Autodesk Inventor part; units mm, degrees
ref_plane "YZ Plane" through (0, 0, 0) normal (1, 0, 0) x (0, 1, 0)
ref_plane "XZ Plane" through (0, 0, 0) normal (0, 1, 0) x (-1, 0, 0)
ref_plane "XY Plane" through (0, 0, 0) normal (0, 0, 1) x (1, 0, 0)
sketch "Sketch1" plane through (0, 0, 0) normal (0, 0, 1) x (1, 0, 0)
  circle A0 centre (0, 0) radius 22.5
extrude "Extrusion1" add sketch "Sketch1" along normal blind 12
sketch "Sketch2" plane through (0, 0, 12) normal (0, 0, 1) x (1, 0, 0)
  circle A0 centre (0, 0) radius 18
extrude "Extrusion2" add sketch "Sketch2" along normal blind 12
sketch "Sketch3" plane through (0, 0, 24) normal (0, 0, 1) x (1, 0, 0)
  circle A0 centre (0, 0) radius 22.5
extrude "Extrusion3" add sketch "Sketch3" along normal blind 20
sketch "Sketch4" plane through (0, 0, 44) normal (0, 0, 1) x (1, 0, 0)
  circle A0 centre (0, 0) radius 35
extrude "Extrusion4" add sketch "Sketch4" along normal blind 36
sketch "Sketch5" plane through (0, 0, 80) normal (0, 0, 1) x (1, 0, 0)
  circle A0 centre (0, 0) radius 25
extrude "Extrusion5" cut sketch "Sketch5" against normal blind 15
sketch "Sketch6" plane through (0, 0, 80) normal (0, 0, 1) x (1, 0, 0)
  circle A0 centre (0, 0) radius 35
  line L0 (0, 0) -> (-32.4578, -13.0955)
  line L1 (0, 0) -> (-32.4578, 13.0955)
  arc A1 (-32.4578, 13.0955) -> (-32.4578, -13.0955) centre (0, 0) ccw
  line L2 (0, 0) -> (27.5699, -21.5615)
  line L3 (0, 0) -> (4.8879, -34.657)
  arc A2 (4.8879, -34.657) -> (27.5699, -21.5615) centre (0, 0) ccw
  line L4 (0, 0) -> (4.8879, 34.657)
  line L5 (0, 0) -> (27.5699, 21.5615)
  arc A3 (27.5699, 21.5615) -> (4.8879, 34.657) centre (0, 0) ccw
  dimension "d17" = 360
extrude "Extrusion6" cut sketch "Sketch6" against normal blind 15 contours L5 L4 A0 | A0 L3 L2 | L0 A0 L1
sketch "Sketch7" plane through (0, 0, 65) normal (0, 0, 1) x (1, 0, 0)
  arc A0 (11.4564, 5) -> (11.4564, -5) centre (0, 0) ccw
  line L0 (18.8783, 0) -> (18.8783, 5)
  line L1 (18.8783, 0) -> (18.8783, -5)
  line L2 (18.8783, -5) -> (11.4564, -5)
  line L3 (18.8783, 5) -> (11.4564, 5)
extrude "Extrusion7" cut sketch "Sketch7" against normal blind 16
sketch "Sketch8" plane through (0, 0, 0) normal (0, 0, -1) x (-1, 0, 0)
  point P0 (0, 0)
sketch "Sketch9" plane through (0, 0, 49) normal (0, 0, 1) x (1, 0, 0)
  circle A0 centre (0, 0) radius 11.9112
extrude "Extrusion8" cut sketch "Sketch9" against normal blind 50.8
properties part number "tarea 3 dinamica" material "Iron, Ductile"
Part model, mm, in its own coordinate system. A direction names the side the tool comes from. Give positions to 0.01 mm unless a question says otherwise; leave off trailing zeros. Loops run counter-clockwise (first coordinate to the right, second up) from the corner with the lowest first, then second, coordinate; pieces in that order, holes last. Notation, with made-up numbers: (73.5, 36.25) -> (126.5, 36.25) arc R18 cw to (126.5, 65.25) -> close; hole circle Ø9 at (-32.5, 88). An arc over 180 degrees is marked (long way). Write each question's results on one line, items separated by ' | '. Start each with the question number.
Q1. Which spindle directions (+Z, -Z, +X, -X, +Y, -Y) get a long thin tool onto all of the face, cutting with end or side? Do faces 1 (the face through (-12.298, 21.766, 72.605)), 2 (the face through (23.58, -18.44, 72.6)), 3 (the face through (4.18, -29.64, 72.6)). Say none if no direction does.
Q2. Band-saw the part on C-C on z = 54. List the corners of the cut face in (x, y).
Q3. Band-saw the part on A-A on x = 0. List the corners of the cut face in (y, z).
Q4. Wall check: L1, parallel to Y at x = 0, z = 56.25; L2, parallel to Z at x = 14, y = -17; L3, parallel to Y at x = 0, z = 20. Give the ranges that are in metal, low to high.
Q5. Pull direction X, two halves, no side cores. Call faces 4 (the face through (10.382, 19.961, 33.86)), 5 (the face through (-10.1, 15.1, 24)), 6 (the face through (12.4, 0.1, 49)), 7 (the face through (4.18, 29.64, 72.6)): +X half, -X half, draft (parallel to the pull), parting line (faces both ways), or undercut.
Q6. Pin check, flat tips, straight feed: P1, Ø21.5, axis at x = 0, y = 0, coming from the +Z side; P2, Ø12, axis at y = 18.5, z = 41.5, coming from the +X side; P3, Ø1, axis at x = 12, z = 49, coming from the +Y side; P4, Ø2, axis at x = 15, z = 56.5, coming from the +Y side. Stop position of each tip, or through.
Q7. Band-saw the part on D-D on z = 69. List the corners of the cut face in (x, y) (1 decimal), plus the area to 3 significant figures.
Q8. Band-saw the part on B-B on y = 0. List the corners of the cut face in (x, z).
Results are:
1) face 1: +Z | face 2: +Z, -Y | face 3: +Z, +X
2) outline: circle Ø70 at (0, 0); hole (11.46, -5) -> (18.88, -5) -> (18.88, 5) -> (11.46, 5) arc R12.5 ccw (long way) to start
3) outline: (-35, 44) -> (-22.5, 44) -> (-22.5, 24) -> (-18, 24) -> (-18, 12) -> (-22.5, 12) -> (-22.5, 0) -> (-11.91, 0) -> (-11.91, 49) -> (-12.5, 49) -> (-12.5, 65) -> (-25, 65) -> (-25, 80) -> (-35, 80) -> close; (11.91, 0) -> (22.5, 0) -> (22.5, 12) -> (18, 12) -> (18, 24) -> (22.5, 24) -> (22.5, 44) -> (35, 44) -> (35, 80) -> (25, 80) -> (25, 65) -> (12.5, 65) -> (12.5, 49) -> (11.91, 49) -> close
4) L1: y = -35 to -12.5, 12.5 to 35 | L2: z = 0 to 12, 24 to 65 | L3: y = -18 to -11.91, 11.91 to 18
5) face 4: parting line | face 5: draft | face 6: undercut | face 7: +X half
6) P1: passes through | P2: stops at x = 32.48 | P3: stops at y = 33.06 | P4: stops at y = 32.08
7) outline: (-32.5, -13.1) arc R35 ccw to (4.9, -34.7) -> (3.5, -24.8) arc R25 cw to (-23.2, -9.4) -> close; (-32.5, 13.1) -> (-23.2, 9.4) arc R25 cw to (3.5, 24.8) -> (4.9, 34.7) arc R35 ccw to start; (19.7, -15.4) -> (27.6, -21.6) arc R35 ccw to (27.6, 21.6) -> (19.7, 15.4) arc R25 cw to start | area: 1,190 mm²
8) outline: (-35, 44) -> (-22.5, 44) -> (-22.5, 24) -> (-18, 24) -> (-18, 12) -> (-22.5, 12) -> (-22.5, 0) -> (-11.91, 0) -> (-11.91, 49) -> (-12.5, 49) -> (-12.5, 65) -> (-35, 65) -> close; (11.91, 0) -> (22.5, 0) -> (22.5, 12) -> (18, 12) -> (18, 24) -> (22.5, 24) -> (22.5, 44) -> (35, 44) -> (35, 80) -> (25, 80) -> (25, 65) -> (18.88, 65) -> (18.88, 49) -> (11.91, 49) -> close
